Can you work these out from the model? Positions are in its coordinate system, mm. A direction names the side the tool comes from. Coordinates: 2 decimals unless noted, no trailing zeros. Order: outer loops, then holes, each group sorted by start corner. A loop starts at its lowest first (then second) coordinate and runs counter-clockwise, first axis right, second up. Notation, with made-up numbers: (47.5, 36) - (80.5, 36) arc R21 cw to (80.5, 49) - close; hole circle Ø4 at (12, 30). An arc over 180 degrees is marked (long way). Return JSON: item names as keys, results as strings. Group by question number.
1) Imagine slicing it at A-A (x = 14.5). Write out the boundary of the cut face in (y, z), and give its area (3 significant figures).
2) Imagine slicing it at B-B (y = 12). Write out the boundary of the cut face in (x, z).
3) Which directions (+Z, -Z, +X, -X, +Y, -Y) give clear straight access to the entire face, cutting with the end or side of a thin tool? Please do faces 1 (the face through (2, 73, -2)), 2 (the face through (17.4, 0.57, 0.99)).
4) For pin 1 Ø10 at (x, y) = (6, 19.5) entering from -Z; pin 2 Ø3 at (y, z) = (71.07, -4) entering from -X, each with a flat end and sliding along its axis, tell me the tip position at first contact or that it passes through.
5) If I drill on line 1 along Z through (x, y) = (7.25, 18); line 2 along Y through (x, z) = (16.75, 1.5); line 3 along Y through (x, z) = (1.5, -0.25), over which ranges is the centre line in solid material (lowest first)?
6) Imagine slicing it at C-C (z = -5). Write out the boundary of the cut face in (x, y).
```python
from build123d import *

# Parameters (mm, degrees)
PAD_DEPTH    = 2
FILLET_R     = 0.5
SKETCH001_R  = 2
PAD001_DEPTH = 2


with BuildPart() as part:
    # Sketch → Pad (new body)
    with BuildSketch(Plane.XY):
        with BuildLine():
            ThreePointArc((0, 2), (0.585786, 0.585786), (2, 0))
            Line((16, 0), (2, 0))
            ThreePointArc((16, 0), (17.414214, 0.585786), (18, 2))
            Line((18, 78), (18, 2))
            ThreePointArc((18, 78), (17.414214, 79.414214), (16, 80))
            Line((2, 80), (16, 80))
            ThreePointArc((2, 80), (0.585786, 79.414214), (0, 78))
            Line((0, 2), (0, 78))
        make_face()
    extrude(amount=PAD_DEPTH)

    # Fillet
    fillet_edges = [part.edges().sort_by_distance(p)[0] for p in [
        (18, 78, 1),
        (18, 2, 1),
        (18, 40, 0),
        (18, 40, 2),
    ]]
    fillet(fillet_edges, radius=FILLET_R)

    # Sketch001 → Pad001 (join)
    with BuildSketch(Plane.YZ):
        with BuildLine():
            Line((78, 0), (64.143594, 0))
            Line((64.143594, 0), (67.607695, -6))
            ThreePointArc((67.607695, -6), (71.071797, -8), (74.535898, -6))
            Line((74.535898, -6), (78, 0))
        make_face()
        with Locations((71.071797, -4)):
            Circle(SKETCH001_R, mode=Mode.SUBTRACT)
    extrude(amount=PAD001_DEPTH)


solid = part.part
```
Calculated:
{
 "1": {"outline": "(0, 0.5) arc R0.5 ccw to (0.5, 0) - (79.5, 0) arc R0.5 ccw to (80, 0.5) - (80, 1.5) arc R0.5 ccw to (79.5, 2) - (0.5, 2) arc R0.5 ccw to (0, 1.5) - close", "area": "160 mm2"},
 "2": {"outline": "(0, 0.5) arc R0.5 ccw to (0.5, 0) - (17.5, 0) arc R0.5 ccw to (18, 0.5) - (18, 1.5) arc R0.5 ccw to (17.5, 2) - (0.5, 2) arc R0.5 ccw to (0, 1.5) - close"},
 "3": {"face 1": "-Z, +X, +Y, -Y", "face 2": "+Z, -Z, +X, -Y"},
 "4": {"pin 1": "z = 0", "pin 2": "through"},
 "5": {"line 1": "0 to 2", "line 2": "0.15 to 79.85", "line 3": "64.29 to 77.86"},
 "6": {"outline": "(0, 67.03) - (2, 67.03) - (2, 69.34) - (0, 69.34) - close; (0, 72.8) - (2, 72.8) - (2, 75.11) - (0, 75.11) - close"}
}
